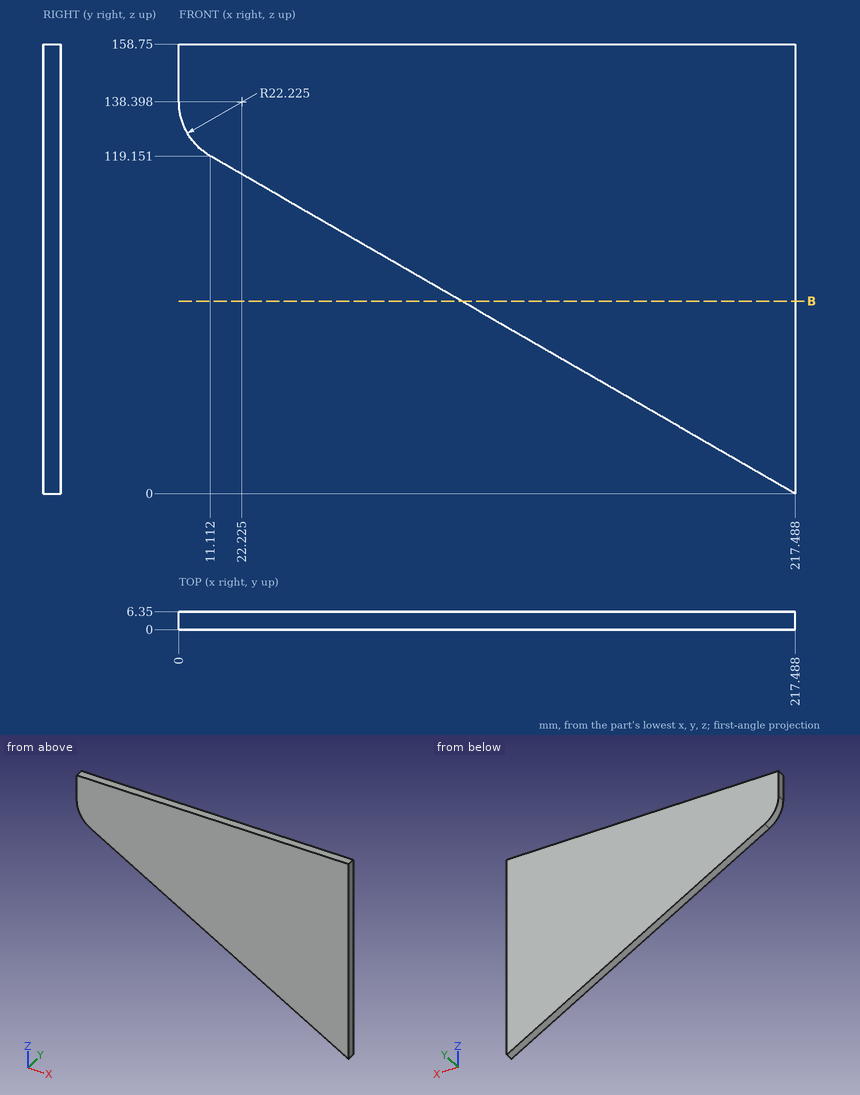
Verification items for this drawing (mm, ordinates from the low corner). Round coordinates to 2 decimals unless told otherwise and drop trailing zeros. Write each loop counter-clockwise with the first axis right and the second up, starting at its lowest first coordinate (ties: lowest second). Pieces come first, ordered by that corner, then holes. Notation, with made-up numbers: (3.25, 82.25) - (14.25, 82.25) arc R17 ccw to (14.25, 95.25) - close; hole circle Ø3 at (-37.75, -19.75). An arc over 180 degrees is marked (long way). Answer as a JSON object with one key per item and string values. Group by question number.
Q1. Thickness scan on line 1 (Z direction, x = 151.5, y = 2.5); line 2 (Z direction, x = 84, y = 2.25); line 3 (X direction, y = 6.25, z = 133.5) (1 decimal). Record the ranges inside material, lowest first.
Q2. Section check B-B, the plane z = 68. Enter the section's corners in (x, y), plus the area to 3 significant figures.
Q3. Go/stop test with flat-tipped pins: pin 1 Ø1 at (x, y) = (40, 3.5) entering from -Z (1 decimal); pin 2 Ø3 at (y, z) = (2, 56.5) entering from -X; pin 3 Ø3 at (y, z) = (3.5, 60) entering from -X (1 decimal). Record where each tip stops, or that it passes through.
Found:
{
 "1": {"line 1": "z = 38.1 to 158.75", "line 2": "z = 77.07 to 158.75", "line 3": "x = 0.5 to 217.5"},
 "2": {"outline": "(99.71, 0) - (217.49, 0) - (217.49, 6.35) - (99.71, 6.35) - close", "area": "748 mm^2"},
 "3": {"pin 1": "stops at z = 102.2", "pin 2": "stops at x = 117.03", "pin 3": "stops at x = 111"}
}
